Verification items for this drawing (mm, ordinates from the low corner). A direction names the side the tool comes from. Give positions to 0.01 mm unless a question says otherwise; leave off trailing zeros. Loops run counter-clockwise (first coordinate to the right, second up) from the corner with the lowest first, then second, coordinate; pieces in that order, holes last. Notation, with made-up numbers: M -7.75,38 L 50.25,38 A13 ccw 50.25,55 Z; hole C -15.5,-37 d11. An arc over 180 degrees is marked long. Use one line per item in the form item = value.
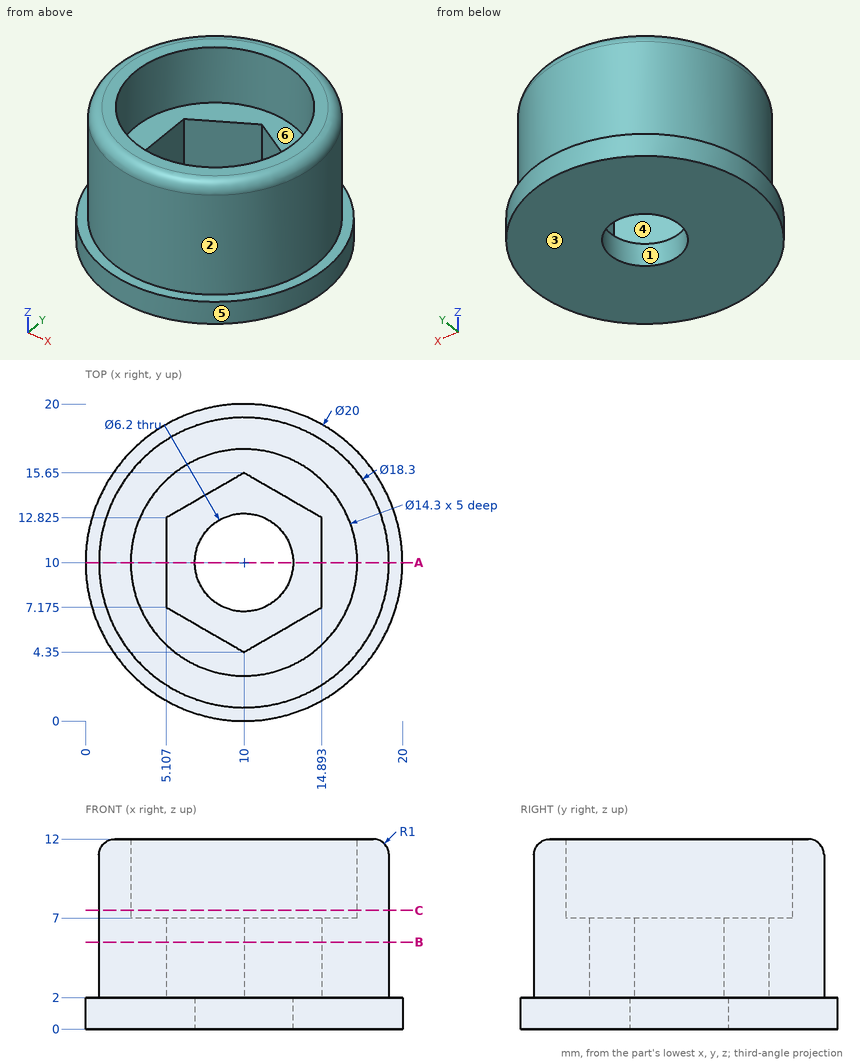
1) Set-up check for the marked faces 1 and 2: record each of +Z, -Z, +X, -X, +Y, -Y from which the full face is reachable in a straight line by a thin tool's end or side.
Evaluation:
face_1 = +Z, -Z
face_2 = +Z
2) Scan lines: line 1 (Y direction, x = 10, z = 1.2); line 2 (Y direction, x = 10, z = 10); line 3 (Z direction, x = 7, y = 18.75). Record each from-to range of solid material in increasing order.
Evaluation:
line_1 = 0 to 6.9, 13.1 to 20
line_2 = 0.85 to 2.85, 17.15 to 19.15
line_3 = 0 to 2
3) Section check B-B (z = 5.5). Record the cut outline in (x, y) (3 decimals).
Evaluation:
outline = C 10,10 d18.3; hole M 5.107,7.175 L 10,4.35 L 14.893,7.175 L 14.893,12.825 L 10,15.65 L 5.107,12.825 Z
4) Depth check by flat-ended pin: pin 1 Ø2.5 at (y, z) = (9, 4.5) entering from +X; pin 2 Ø2 at (x, z) = (17.5, 1.5) entering from +Y; pin 3 Ø10 at (x, y) = (10, 10) entering from +Z. Enter the tip coordinate at first touch or a pass-through.
Evaluation:
pin_1 = 19.15
pin_2 = 17.6
pin_3 = 7
5) Section check C-C (z = 7.5). Record the cut outline in (x, y), then the cut area to 3 significant figures.
Evaluation:
outline = C 10,10 d18.3; hole C 10,10 d14.3
area = 102 mm^2
6) Release check for a two-part mould opening along Y. For the marked faces 3, 4, 5 and 6 record: pulls with the +Y half, pulls with the -Y half, needs draft (parallel to the pull), parting line crosses it, or undercut.
Evaluation:
face_3 = needs draft
face_4 = undercut
face_5 = parting line crosses it
face_6 = undercut
7) Section check A-A (y = 10). Record the cut outline in (x, z), then the cut area to 3 significant figures.
Evaluation:
outline = M 0,0 L 6.9,0 L 6.9,2 L 5.11,2 L 5.11,7 L 2.85,7 L 2.85,12 L 1.85,12 A1 ccw 0.85,11 L 0.85,2 L 0,2 Z; M 13.1,0 L 20,0 L 20,2 L 19.15,2 L 19.15,11 A1 ccw 18.15,12 L 17.15,12 L 17.15,7 L 14.89,7 L 14.89,2 L 13.1,2 Z
area = 89.7 mm^2
